Geometry check sheet. Reference: drawing and pictorial views, mm from the part's lowest x, y, z. A direction names the side the tool comes from. Round coordinates to 2 decimals unless told otherwise and drop trailing zeros. Loops run counter-clockwise (first coordinate to the right, second up) from the corner with the lowest first, then second, coordinate; pieces in that order, holes last. Notation, with made-up numbers: (78, 20.25) -> (108, 20.25) arc R29 cw to (108, 54.25) -> close; hole circle Ø3 at (63.5, 1.5). An arc over 180 degrees is marked (long way). Use one line per item in the form item = value. Start each with the question number.
(1) Sectioned sample at B-B (y = 10.5). Record the cut outline in (x, z).
(2) Draft check along X on the marked faces 3, 4, 5 and 6. Enter one of: released by +X, released by -X, zero draft, split by the parting line, or undercut.
(3) Go/stop test with flat-tipped pins: pin 1 (0.5 mm diameter, centred on x = 0.5, y = 14.5, fed in from -Z); pin 2 (1.2 mm diameter, centred on x = 19, y = 40.5, fed in from -Z); pin 3 (5.5 mm diameter, centred on x = 30.5, z = 7.5, fed in from +Y). Record where each tip stops, or that it passes through.
(4) Sectioned sample at D-D (z = 10.75). Record the cut outline in (x, y), and give its area (3 significant figures).
(5) Material ranges on probe 1 along Y at (x, z) = (15.5, 15); probe 2 along X at (y, z) = (5, 2); probe 3 along Y at (x, z) = (50.5, 6.5), recorded low to high. Write a range as [from, to].
(6) Set-up check for the marked faces 1 and 2: record each of +Z, -Z, +X, -X, +Y, -Y from which the full face is reachable in a straight line by a thin tool's end or side.
(7) Sectioned sample at C-C (x = 17). Record the cut outline in (y, z).
(8) Sectioned sample at A-A (z = 5.25). State how many separate pieces and enclosed holes the cut face has.
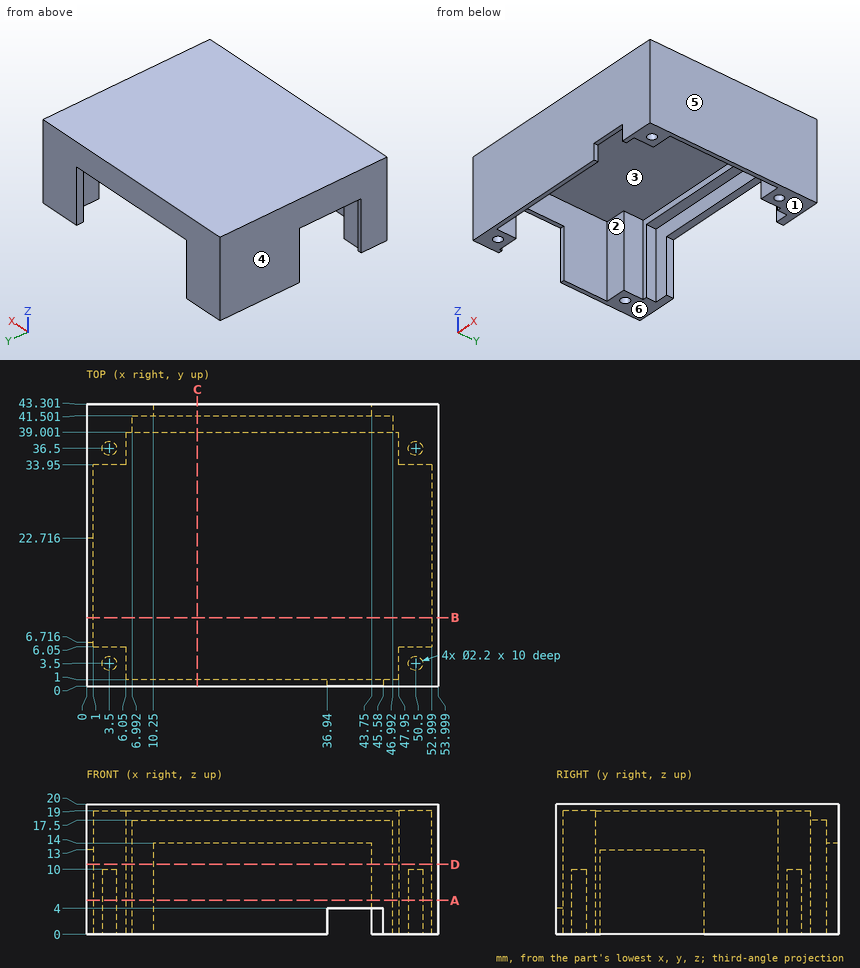
Checks:
q1.outline = (0, 13) -> (1, 13) -> (1, 19) -> (53, 19) -> (53, 0) -> (54, 0) -> (54, 20) -> (0, 20) -> close
q2.face_3 = undercut
q2.face_4 = released by -X
q2.face_5 = released by +X
q2.face_6 = zero draft
q3.pin_1 = 13
q3.pin_2 = 17.5
q3.pin_3 = 1
q4.outline = (0, 0) -> (54, 0) -> (54, 43.3) -> (43.75, 43.3) -> (43.75, 41.5) -> (46.99, 41.5) -> (46.99, 39) -> (47.95, 39) -> (47.95, 33.95) -> (53, 33.95) -> (53, 6.05) -> (47.95, 6.05) -> (47.95, 1) -> (6.05, 1) -> (6.05, 6.05) -> (1, 6.05) -> (1, 6.72) -> (0, 6.72) -> close; (0, 22.72) -> (1, 22.72) -> (1, 33.95) -> (6.05, 33.95) -> (6.05, 39) -> (6.99, 39) -> (6.99, 41.5) -> (10.25, 41.5) -> (10.25, 43.3) -> (0, 43.3) -> close
q4.area = 288 mm2
q5.probe_1 = [0, 1], [41.5, 43.3]
q5.probe_2 = [0, 6.05], [47.95, 54]
q5.probe_3 = [0, 2.4], [4.6, 6.05], [33.95, 35.4], [37.6, 43.3]
q6.face_1 = -Z, +X, -X, +Y, -Y
q6.face_2 = -Z
q7.outline = (0, 0) -> (1, 0) -> (1, 19) -> (39, 19) -> (39, 17.5) -> (41.5, 17.5) -> (41.5, 14) -> (43.3, 14) -> (43.3, 20) -> (0, 20) -> close
q8.separate_pieces = 2
q8.enclosed_holes = 4
